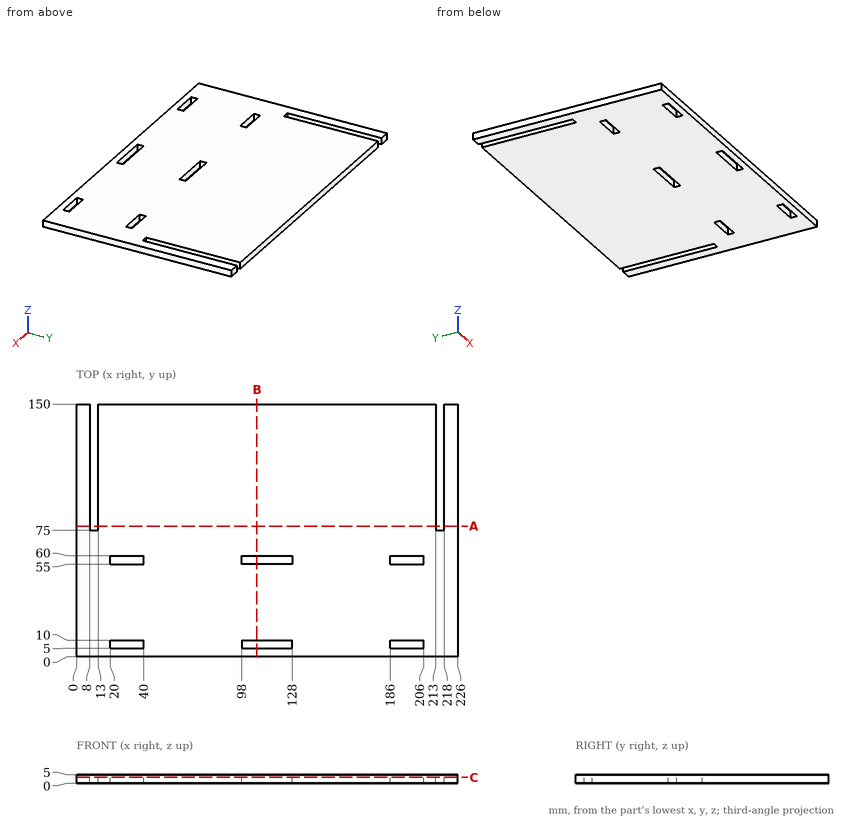
Geometry check sheet. Reference: drawing and pictorial views, mm from the part's lowest x, y, z. Round coordinates to 2 decimals unless told otherwise and drop trailing zeros. Write each loop counter-clockwise with the first axis right and the second up, starting at its lowest first coordinate (ties: lowest second). Pieces come first, ordered by that corner, then holes.
1. Gauge pin test, flat end, axial feed: P1, Ø1.5, axis at x = 10, z = 1.5, coming from the +Y side. Record the tip position at first contact, or that the pin passes through.
2. Section check A-A on y = 77.5. Enter the section's corners in (x, z).
3. Scan lines: L1, parallel to X at y = 106.5, z = 4.7; L2, parallel to Y at x = 190, z = 1.6; L3, parallel to X at y = 57.5, z = 4.05. Record each from-to range of solid material in increasing order.
4. Section check B-B on x = 107. Enter the section's corners in (y, z).
5. Section check C-C on z = 3.5. State how many separate pieces and enclosed holes the cut face has, plus the area to 4 significant figures.
Answer:
1. P1: stops at y = 75
2. outline: (0, 0) - (8, 0) - (8, 5) - (0, 5) - close; (13, 0) - (213, 0) - (213, 5) - (13, 5) - close; (218, 0) - (226, 0) - (226, 5) - (218, 5) - close
3. L1: x = 0 to 8, 13 to 213, 218 to 226
3. L2: y = 0 to 5, 10 to 55, 60 to 150
3. L3: x = 0 to 20, 40 to 98, 128 to 186, 206 to 226
4. outline: (0, 0) - (5, 0) - (5, 5) - (0, 5) - close; (10, 0) - (55, 0) - (55, 5) - (10, 5) - close; (60, 0) - (150, 0) - (150, 5) - (60, 5) - close
5. separate pieces: 1
5. enclosed holes: 6
5. area: 32,450 mm2
